For this review, take the finished solid that the model builds, in its own axes (mm). A direction names the side the tool comes from. Coordinates: 2 decimals unless noted, no trailing zeros. Order: outer loops, then holes, each group sorted by start corner. A loop starts at its lowest first (then second) coordinate and runs counter-clockwise, first axis right, second up. Notation, with made-up numbers: M -31.75,38.25 L 9.25,38.25 A24 cw 9.25,65.25 Z; hole C -2.5,-24.5 d5. An arc over 180 degrees is marked long. Use CSV: the item, a comma, the result in double quotes.
```python
from build123d import *

# Parameters (mm, degrees)
ESBO_O1_W                = 30
ESBO_O1_H                = 5
RESSALTO_EXTRUS_O1_DEPTH = 1.5
ESBO_O2_W                = 2
ESBO_O2_H                = 5
RESSALTO_EXTRUS_O2_DEPTH = 7
FILETE1_R                = 2
FILETE2_R                = 2
CHANFRO1_SIZE            = 2
FILETE4_R                = 0.5
FILETE5_R                = 0.5


with BuildPart() as part:
    # Esboço1 → Ressalto-extrusão1 (new body)
    with BuildSketch(Plane(origin=(0, 0, 0), x_dir=(1, 0, 0), z_dir=(0, 1, 0))):
        Rectangle(ESBO_O1_W, ESBO_O1_H)
    extrude(amount=RESSALTO_EXTRUS_O1_DEPTH)

    # Esboço2 → Ressalto-extrusão2 (add)
    with BuildSketch(Plane(origin=(0, 1.5, 0), x_dir=(1, 0, 0), z_dir=(0, 1, 0))):
        with Locations((14, 0)):
            Rectangle(ESBO_O2_W, ESBO_O2_H)
    extrude(amount=RESSALTO_EXTRUS_O2_DEPTH)

    # Filete1
    filete1_edges = [part.edges().sort_by_distance(p)[0] for p in [
        (-15, 0.75, 2.5),
    ]]
    fillet(filete1_edges, radius=FILETE1_R)

    # Filete2
    filete2_edges = [part.edges().sort_by_distance(p)[0] for p in [
        (-15, 0.75, -2.5),
    ]]
    fillet(filete2_edges, radius=FILETE2_R)

    # Chanfro1
    chanfro1_edges = [part.edges().sort_by_distance(p)[0] for p in [
        (13, 1.5, 0),
    ]]
    chamfer(chanfro1_edges, length=CHANFRO1_SIZE)

    # Filete4
    filete4_edges = [part.edges().sort_by_distance(p)[0] for p in [
        (13, 6, 2.5),
    ]]
    fillet(filete4_edges, radius=FILETE4_R)

    # Filete5
    filete5_edges = [part.edges().sort_by_distance(p)[0] for p in [
        (13, 6, -2.5),
    ]]
    fillet(filete5_edges, radius=FILETE5_R)


solid = part.part
```
Item 1: For faces 1 (the face through (-2, 1.5, 0)), 2 (the face through (0, 0, 0)), list the 3-axis set-ups (+Z, -Z, +X, -X, +Y, -Y) from which the entire face can be reached by the end or side of a thin tool; tool diameter is ignored.
Solutions:
face 1,"+Z, -Z, -X, +Y"
face 2,"+Z, -Z, +X, -X, -Y"
Item 2: Add section A-A on z = -0.15. State the section outline as (x, y) points, and give its area (3 significant figures).
Solutions:
outline,"M -15,0 L 15,0 L 15,8.5 L 13,8.5 L 13,3.5 L 11,1.5 L -15,1.5 Z"
area,"61.0 mm^2"
Item 3: To check wall thickness, follow line 1 along X through (y, z) = (6, -0.1); line 2 along Y through (x, z) = (8.75, -1.45); line 3 along X through (y, z) = (3.25, 1.1). State the ranges of each line that lie inside material, in increasing order. Write a range as [from, to].
Solutions:
line 1,"[13, 15]"
line 2,"[0, 1.5]"
line 3,"[12.75, 15]"
Item 4: Add section C-C on x = -0.5. State the section outline as (y, z) points.
Solutions:
outline,"M 0,-2.5 L 1.5,-2.5 L 1.5,2.5 L 0,2.5 Z"
Item 5: Add section D-D on z = 1.15. State the section outline as (x, y) points, and give its area (3 significant figures).
Solutions:
outline,"M -14.89,0 L 15,0 L 15,8.5 L 13,8.5 L 13,3.5 L 11,1.5 L -14.89,1.5 Z"
area,"60.8 mm^2"
Item 6: Add section B-B on y = 5.5. State the section outline as (x, z) points, and give its area (3 significant figures).
Solutions:
outline,"M 13,-2 A0.5 ccw 13.5,-2.5 L 15,-2.5 L 15,2.5 L 13.5,2.5 A0.5 ccw 13,2 Z"
area,"9.89 mm^2"
Item 7: Clearance check with a flat-ended pin moving along its axis: pin 1 Ø1.2 at (y, z) = (7, -1) entering from -X. State where the tip first meets the part, or that it passes through.
Solutions:
pin 1,"x = 13"
